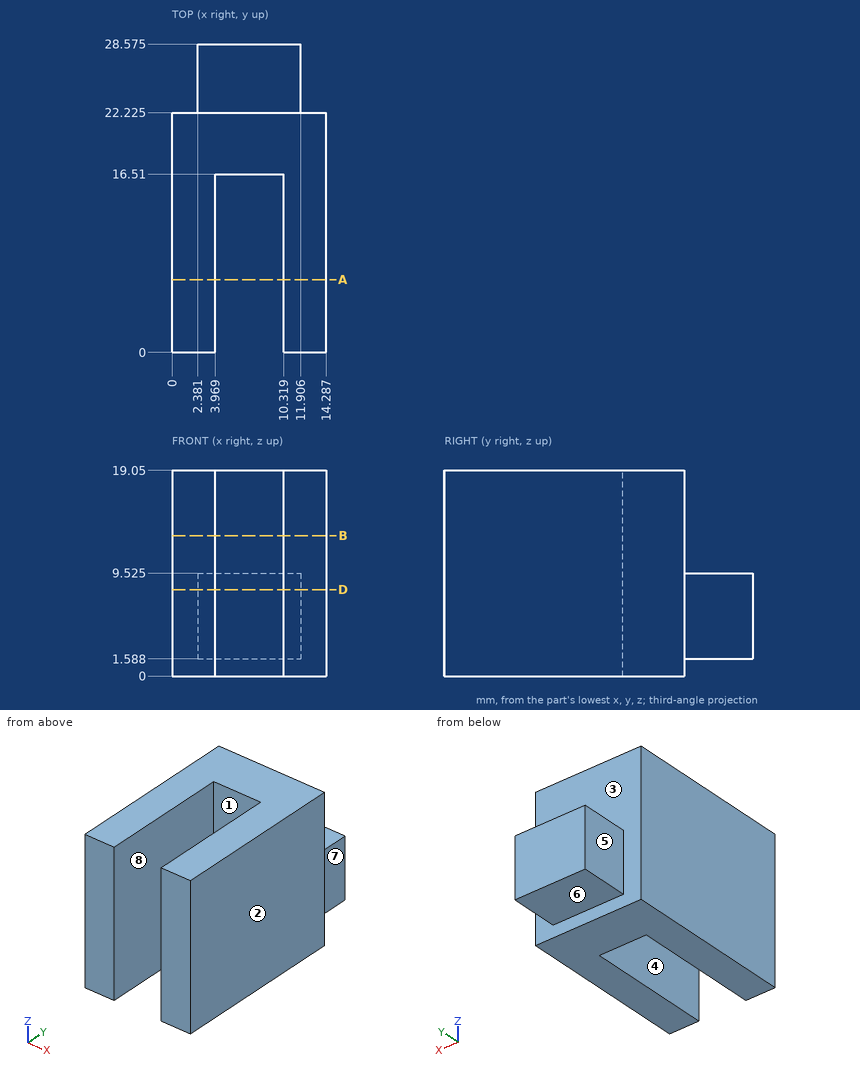
For this review, use the dimensioned drawing (mm, ordinates from the lowest corner) and the shaded views. A direction names the side the tool comes from. Round coordinates to 2 decimals unless told otherwise and drop trailing zeros. Order: outer loops, then holes, each group sorted by start corner. A loop starts at its lowest first (then second) coordinate and runs counter-clockwise, first axis right, second up. Notation, with made-up numbers: (4, 31.25) -> (46, 31.25) arc R32 cw to (46, 70.25) -> close; hole circle Ø5 at (51, 55). An arc over 180 degrees is marked (long way). Put each result on its own line as item: value.
Q1. Mouldability with a two-part tool opening along X and no side actions: class the marked faces 1, 2, 3 and 4 as pulls with the +X half, pulls with the -X half, needs draft (parallel to the pull), parting line crosses it, or undercut.
Check result:
face 1: undercut
face 2: pulls with the +X half
face 3: needs draft
face 4: undercut
Q2. Add section B-B on z = 13. Write out the cut boundary in (x, y) (1 decimal).
Check result:
outline: (0, 0) -> (4, 0) -> (4, 16.5) -> (10.3, 16.5) -> (10.3, 0) -> (14.3, 0) -> (14.3, 22.2) -> (0, 22.2) -> close
Q3. Machinability: for the marked faces 5, 6, 7 and 8, which of the approach directions +Z, -Z, +X, -X, +Y, -Y give a long, thin tool a straight path to every point of the face, cutting with its end or side? Answer none if there is none.
Check result:
face 5: +Z, -Z, -X, +Y
face 6: -Z, +X, -X, +Y
face 7: +Z, -Z, +X, +Y
face 8: +Z, -Z, -Y
Q4. Add section A-A on y = 6.75. Write out the cut boundary in (x, z), plus the area to 3 significant figures.
Check result:
outline: (0, 0) -> (3.97, 0) -> (3.97, 19.05) -> (0, 19.05) -> close; (10.32, 0) -> (14.29, 0) -> (14.29, 19.05) -> (10.32, 19.05) -> close
area: 151 mm2
Q5. Add section D-D on z = 8. Write out the cut boundary in (x, y) (1 decimal), plus the area to 3 significant figures.
Check result:
outline: (0, 0) -> (4, 0) -> (4, 16.5) -> (10.3, 16.5) -> (10.3, 0) -> (14.3, 0) -> (14.3, 22.2) -> (11.9, 22.2) -> (11.9, 28.6) -> (2.4, 28.6) -> (2.4, 22.2) -> (0, 22.2) -> close
area: 273 mm2
Q6. For probe 1 along X at (y, z) = (13.75, 4.5); probe 2 along X at (y, z) = (25, 8); probe 3 along Y at (x, z) = (6.75, 17.75) (1 decimal), list the stretches that pass through material, from the lowest coordinate up. Write a range as [from, to].
Check result:
probe 1: [0, 3.97], [10.32, 14.29]
probe 2: [2.38, 11.91]
probe 3: [16.5, 22.2]
Q7. Insertion check: pin 1 Ø1.9 at (y, z) = (26, 6) entering from +X; pin 2 Ø7 at (x, y) = (7.5, 26.5) entering from +Z (1 decimal); pin 3 Ø4.5 at (x, z) = (6.5, 13.5) entering from +Y (1 decimal). Each pin has a flat end and moves straight along its axis. Give the tip position at first contact, or say it passes through.
Check result:
pin 1: x = 11.91
pin 2: z = 9.5
pin 3: y = 22.2
